Verification items for the finished model (mm, model axes). A direction names the side the tool comes from. Coordinates: 2 decimals unless noted, no trailing zeros. Order: outer loops, then holes, each group sorted by start corner. A loop starts at its lowest first (then second) coordinate and runs counter-clockwise, first axis right, second up.
Q1. Draft check along Y on faces 3 (the flat face through (51, -19.05, 6)), 4 (the flat face through (19, -15, 38.1)), 5 (the flat face through (31, -25.4, 11)). Enter one of: pulls with the +Y half, pulls with the -Y half, needs draft (parallel to the pull), parting line crosses it, or undercut.
Q2. Cross-section at A-A, the plane x = 61. Record the boundary of the cut face in (y, z).
Q3. Cross-section at C-C, the plane z = 8. Record the boundary of the cut face in (x, y), and give its area (3 significant figures).
Q4. Depth check by flat-ended pin: P1, Ø10, axis at x = 26, y = -15.5, coming from the -Z side; P2, Ø6, axis at x = 42, y = -22.5, coming from the +Z side; P3, Ø2, axis at y = -5.5, z = 13.5, coming from the -X side; P4, Ø7.5, axis at x = 12.7, y = -12.84, coming from the -Z side. Enter the tip coordinate at first touch or a pass-through.
Q5. Cross-section at D-D, the plane y = -5.25. Record the boundary of the cut face in (x, z), and give its area (3 significant figures).
Q6. Cross-section at B-B, the plane y = -13.75. Record the boundary of the cut face in (x, z).
Q7. Set-up check for faces 1 (the flat face through (51, -6.35, 6)), 2 (the cylindrical face through (76.08, -12.42, 6.44)): record each of +Z, -Z, +X, -X, +Y, -Y from which the full face is reachable in a straight line by a thin tool's end or side.
Q8. Thickness scan on line 1 (Y direction, x = 12.7, z = 27); line 2 (X direction, y = -12.5, z = 28); line 3 (X direction, y = -8, z = 3). Record the ranges inside material, lowest first.
from build123d import *

# Parameters (mm, degrees)
F1_DEPTH = 25.4
F3_DEPTH = 25.4
F5_DEPTH = 38.1
F7_DEPTH = 12.7
F8_R     = 6.35
F9_DEPTH = 38.1


with BuildPart() as f1:
    # F0 (on Front) → F1 (new body)
    with BuildSketch(Plane.XZ):
        Polygon((0, 38.1), (0, 0), (76.2, 0), (76.2, 12.7), (25.4, 12.7), (25.4, 38.1), align=None)
    extrude(amount=F1_DEPTH)

    # F2 (on face) → F3 (cut)
    with BuildSketch(Plane.XY.offset(38.1)):
        with BuildLine():
            ThreePointArc((0, -12.8449322656), (12.7, -0.1449322656), (25.4, -12.8449322656))
            Line((25.4, -12.8449322656), (25.4, 0))
            Line((25.4, 0), (0, 0))
            Line((0, 0), (0, -12.8449322656))
        make_face()
        with BuildLine():
            Line((25.4, -25.4), (25.4, -12.8449322656))
            ThreePointArc((25.4, -12.8449322656), (22.3329497214, -21.1211801875), (14.6131843048, -25.4))
            Line((14.6131843048, -25.4), (25.4, -25.4))
        make_face()
    extrude(amount=-F3_DEPTH, mode=Mode.SUBTRACT)

    # F4 (on face) → F5 (cut)
    with BuildSketch(Plane.XY.offset(38.1)):
        with BuildLine():
            ThreePointArc((0, -12.8449322656), (3.7197438789, -3.8646761445), (12.7, -0.1449322656))
            Line((12.7, -0.1449322656), (0, 0))
            Line((0, 0), (0, -12.8449322656))
        make_face()
        with BuildLine():
            ThreePointArc((10.7868156952, -25.4), (3.0670502786, -21.1211801875), (0, -12.8449322656))
            Line((0, -12.8449322656), (0, -25.4))
            Line((0, -25.4), (10.7868156952, -25.4))
        make_face()
    extrude(amount=-F5_DEPTH, mode=Mode.SUBTRACT)

    # F6 (on face) → F7 (cut)
    with BuildSketch(Plane.XY.offset(12.7)):
        with BuildLine():
            ThreePointArc((44.4495865053, -12.7), (42.5897145658, -8.2098719395), (38.0995865053, -6.35))
            ThreePointArc((38.0995865053, -6.35), (31.7495865053, -12.7), (38.0995865053, -19.05))
            ThreePointArc((38.0995865053, -19.05), (42.5897145658, -17.1901280605), (44.4495865053, -12.7))
        make_face()
        with BuildLine():
            ThreePointArc((63.5, -19.05), (57.15, -12.7), (63.5, -6.35))
            Line((63.5, -6.35), (38.0995865053, -6.35))
            ThreePointArc((38.0995865053, -6.35), (42.5897145658, -8.2098719395), (44.4495865053, -12.7))
            ThreePointArc((44.4495865053, -12.7), (42.5897145658, -17.1901280605), (38.0995865053, -19.05))
            Line((38.0995865053, -19.05), (63.5, -19.05))
        make_face()
        with BuildLine():
            ThreePointArc((63.5, -19.05), (67.9901280605, -17.1901280605), (69.85, -12.7))
            ThreePointArc((69.85, -12.7), (67.9901280605, -8.2098719395), (63.5, -6.35))
            ThreePointArc((63.5, -6.35), (57.15, -12.7), (63.5, -19.05))
        make_face()
        with BuildLine():
            ThreePointArc((63.5, 0), (76.0816873659, -12.7), (63.5, -25.4))
            Line((63.5, -25.4), (76.2, -25.4))
            Line((76.2, -25.4), (76.2, 0))
            Line((76.2, 0), (63.5, 0))
        make_face()
    extrude(amount=-F7_DEPTH, mode=Mode.SUBTRACT)

    # F8 (on face) → F9 (cut)
    with BuildSketch(Plane.XY.offset(38.1)):
        with Locations((12.7, -12.8449322656)):
            Circle(F8_R)
    extrude(amount=-F9_DEPTH, mode=Mode.SUBTRACT)


solid = f1.part
Check values:
1. face 3: undercut
1. face 4: needs draft
1. face 5: pulls with the -Y half
2. outline: (-25.4, 0) - (-19.05, 0) - (-19.05, 12.7) - (-25.4, 12.7) - close; (-6.35, 0) - (0, 0) - (0, 12.7) - (-6.35, 12.7) - close
3. outline: (0, 0) - (12.7, -0.14) arc R12.7 ccw to (10.79, -25.4) - (63.5, -25.4) arc R12.7 ccw to (63.5, 0) - close; hole circle Ø12.7 at (12.7, -12.84); hole (38.1, -19.05) - (63.5, -19.05) arc R6.35 ccw to (63.5, -6.35) - (38.1, -6.35) arc R6.35 ccw to start
3. area: 1,220 mm2
4. P1: stops at z = 0
4. P2: stops at z = 12.7
4. P3: stops at x = 1.7
4. P4: passes through
5. outline: (2.52, 0) - (73.67, 0) - (73.67, 12.7) - (22.88, 12.7) - (22.88, 38.1) - (2.52, 38.1) - close
5. area: 1,420 mm2
6. outline: (0.03, 0) - (6.41, 0) - (6.41, 38.1) - (0.03, 38.1) - close; (18.99, 0) - (31.84, 0) - (31.84, 12.7) - (25.37, 12.7) - (25.37, 38.1) - (18.99, 38.1) - close; (69.76, 0) - (76.04, 0) - (76.04, 12.7) - (69.76, 12.7) - close
7. face 1: +Z, -Z
7. face 2: +Z, -Z, +X
8. line 1: y = -25.4 to -19.19, -6.49 to -0.14
8. line 2: x = 0 to 6.36, 19.04 to 25.4
8. line 3: x = 0.96 to 8.6, 16.8 to 33.83, 67.77 to 75.18
